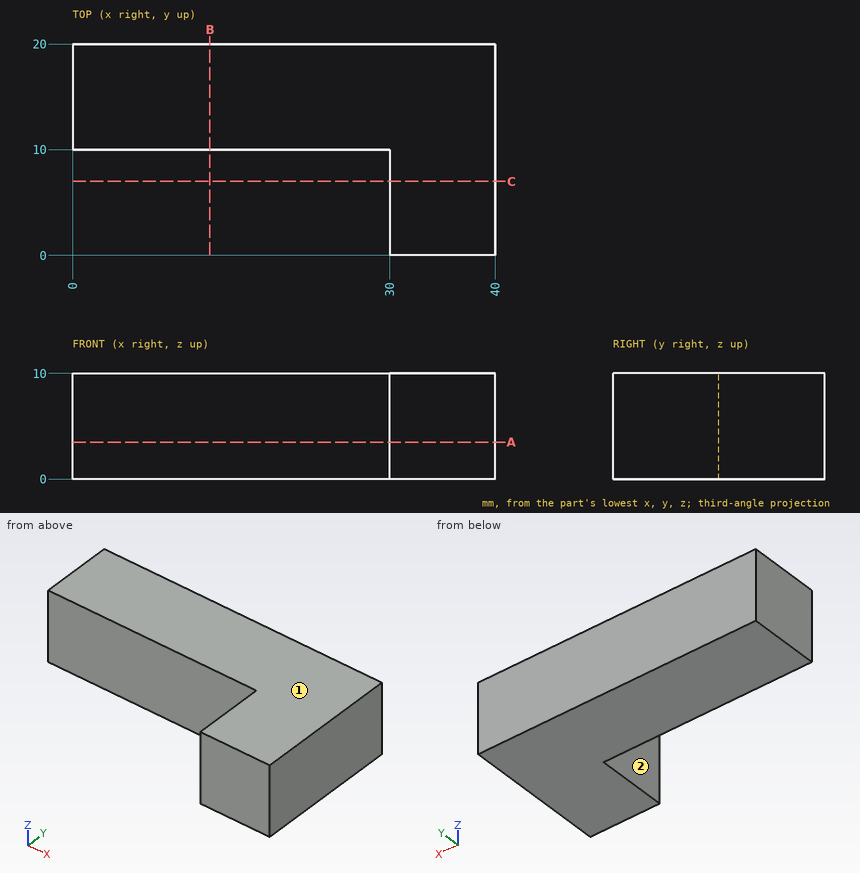
Could you check a few things on this drawing? It's one solid part, dimensions in mm from its lowest x, y, z. A direction names the side the tool comes from. Round coordinates to 2 decimals unless told otherwise and drop trailing zeros. Order: outer loops, then holes, each group sorted by start corner. A loop starts at its lowest first (then second) coordinate and runs counter-clockwise, first axis right, second up.
Q1. Imagine slicing it at C-C, the plane y = 7. List the corners of the cut face in (x, z) for me.
Geometry says:
outline: (30, 0) - (40, 0) - (40, 10) - (30, 10) - close
Q2. Imagine slicing it at A-A, the plane z = 3.5. List the corners of the cut face in (x, y) for me, then the cut area to 3 significant figures.
Geometry says:
outline: (0, 10) - (30, 10) - (30, 0) - (40, 0) - (40, 20) - (0, 20) - close
area: 500 mm2
Q3. Imagine slicing it at B-B, the plane x = 13. List the corners of the cut face in (y, z) for me.
Geometry says:
outline: (10, 0) - (20, 0) - (20, 10) - (10, 10) - close
Q4. I'm going to push flat-ended pins straight in: P1, Ø2, axis at x = 4.5, y = 7.5, coming from the -Z side; P2, Ø2, axis at x = 22, z = 5, coming from the -Y side. Where does each tip first touch, or does it pass through?
Geometry says:
P1: passes through
P2: stops at y = 10
Q5. Please list where these lines run through material, in increasing order: probe 1 along Y at (x, z) = (17.5, 4.5); probe 2 along X at (y, z) = (1, 7.25).
Geometry says:
probe 1: y = 10 to 20
probe 2: x = 30 to 40
Q6. Which directions (+Z, -Z, +X, -X, +Y, -Y) give clear straight access to the entire face, cutting with the end or side of a thin tool? Please do the marked faces 1 and 2.
Geometry says:
face 1: +Z, +X, -X, +Y, -Y
face 2: +Z, -Z, -X, -Y
